For this review, take the finished solid that the model builds, in its own axes (mm). A direction names the side the tool comes from. Coordinates: 2 decimals unless noted, no trailing zeros.
from build123d import *

# Parameters (mm, degrees)
F1_DEPTH     = 7
F2_T2_ANGLE  = 96.7405372454
F2_T4_ANGLE  = 266.8582437325
F2_T6_ANGLE  = 95.969109219
F2_T8_ANGLE  = 264.3512540772
F2_T10_ANGLE = 268.0965177518
F2_T12_ANGLE = 96.2209043171
F2_T14_ANGLE = 96.2209043171
F2_T16_ANGLE = 264.3512540772
F2_T18_ANGLE = 95.969109219
F2_T20_ANGLE = 266.8582437325
F2_T22_ANGLE = 96.7405372454
F2_T24_ANGLE = 268.0965177518


# Not quite as in the source:
# - a fillet or chamfer that OpenCascade refuses, or shapes differently, is made with other operations: its cross-section is extruded or revolved along the edge and cut away or added


with BuildPart() as f1:
    # F0 (on Front) → F1 (new body)
    with BuildSketch(Plane.XZ):
        with BuildLine():
            Line((-28.60048896, 16.5125), (-32.04293994, 18.5))
            ThreePointArc((-32.04293994, 18.5), (-36.2110940276, 7.5997808734), (-36.7769641036, -4.0564653732))
            ThreePointArc((-36.7769641036, -4.0564653732), (-33.6399342951, -1.6712337769), (-29.9995629467, -0.1619351868))
            ThreePointArc((-29.9995629467, -0.1619351868), (-29.5180509711, 5.3558068364), (-28.030388979, 10.6909912395))
            ThreePointArc((-28.030388979, 10.6909912395), (-29.2497876853, 13.5102449097), (-28.60048896, 16.5125))
        make_face()
        with BuildLine():
            ThreePointArc((-28.030388979, 10.6909912395), (-29.5180509711, 5.3558068364), (-29.9995629467, -0.1619351868))
            ThreePointArc((-29.9995629467, -0.1619351868), (-20.1170678219, -0.7895806962), (-12.6676409298, -7.3136659008))
            Line((-12.6676409298, -7.3136659008), (-9.5479300767, -5.5125))
            ThreePointArc((-9.5479300767, -5.5125), (-11.025, 0), (-9.5479300767, 5.5125))
            Line((-9.5479300767, 5.5125), (-19.8969336519, 11.4875))
            ThreePointArc((-19.8969336519, 11.4875), (-23.7589562157, 8.9989236207), (-28.030388979, 10.6909912395))
        make_face()
        with BuildLine():
            ThreePointArc((0, 14.7547752324), (-9.310283358, 17.9279039927), (-14.7448970108, 26.1263853631))
            ThreePointArc((-14.7448970108, 26.1263853631), (-19.3469694385, 22.9280346638), (-23.2738644946, 18.9295333141))
            ThreePointArc((-23.2738644946, 18.9295333141), (-20.3661071395, 17.1899858756), (-19.223711306, 14))
            ThreePointArc((-19.223711306, 14), (-19.3949340289, 12.6994342984), (-19.8969336519, 11.4875))
            Line((-19.8969336519, 11.4875), (-9.5479300767, 5.5125))
            ThreePointArc((-9.5479300767, 5.5125), (-5.5125, 9.5479300767), (0, 11.025))
            Line((0, 11.025), (0, 14.7547752324))
        make_face()
        with BuildLine():
            ThreePointArc((-14.7448970108, 26.1263853631), (-15.2451824532, 30.0359191128), (-14.726480194, 33.9430520298))
            ThreePointArc((-14.726480194, 33.9430520298), (-24.6265431784, 27.6140067915), (-32.04293994, 18.5))
            Line((-32.04293994, 18.5), (-28.60048896, 16.5125))
            ThreePointArc((-28.60048896, 16.5125), (-26.3251091458, 18.5759367359), (-23.2738644946, 18.9295333141))
            ThreePointArc((-23.2738644946, 18.9295333141), (-19.3469694385, 22.9280346638), (-14.7448970108, 26.1263853631))
        make_face()
        with BuildLine():
            ThreePointArc((19.8969336519, 11.4875), (19.6727745701, 16.0763978398), (23.2738644946, 18.9295333141))
            ThreePointArc((23.2738644946, 18.9295333141), (19.3469694385, 22.9280346638), (14.7448970108, 26.1263853631))
            ThreePointArc((14.7448970108, 26.1263853631), (9.310283358, 17.9279039927), (0, 14.7547752324))
            Line((0, 14.7547752324), (0, 11.025))
            ThreePointArc((0, 11.025), (5.5125, 9.5479300767), (9.5479300767, 5.5125))
            Line((9.5479300767, 5.5125), (19.8969336519, 11.4875))
        make_face()
        with BuildLine():
            Line((28.60048896, 16.5125), (32.04293994, 18.5))
            ThreePointArc((32.04293994, 18.5), (24.6265431784, 27.6140067915), (14.726480194, 33.9430520298))
            ThreePointArc((14.726480194, 33.9430520298), (15.1149822826, 31.9885142218), (15.2452247676, 30))
            ThreePointArc((15.2452247676, 30), (15.1196254471, 28.0471035473), (14.7448970108, 26.1263853631))
            ThreePointArc((14.7448970108, 26.1263853631), (19.3469694385, 22.9280346638), (23.2738644946, 18.9295333141))
            ThreePointArc((23.2738644946, 18.9295333141), (26.3251091458, 18.5759367359), (28.60048896, 16.5125))
        make_face()
        with BuildLine():
            ThreePointArc((36.8122346311, -3.7228190211), (36.9530288431, -1.8637755563), (37, 0))
            ThreePointArc((37, 0), (35.7392555727, 9.5763046688), (32.04293994, 18.5))
            Line((32.04293994, 18.5), (28.60048896, 16.5125))
            ThreePointArc((28.60048896, 16.5125), (29.1024885831, 15.3005657016), (29.273711306, 14))
            ThreePointArc((29.273711306, 14), (28.9526221952, 12.2325590968), (28.030388979, 10.6909912395))
            ThreePointArc((28.030388979, 10.6909912395), (29.4933804082, 5.4900375314), (29.9997945679, 0.1110219992))
            ThreePointArc((29.9997945679, 0.1110219992), (33.6494620505, -1.3733111503), (36.8122346311, -3.7228190211))
        make_face()
        with BuildLine():
            ThreePointArc((12.4392811828, -7.1818223394), (19.983625223, -0.5594336383), (29.9997945679, 0.1110219992))
            ThreePointArc((29.9997945679, 0.1110219992), (29.4933804082, 5.4900375314), (28.030388979, 10.6909912395))
            ThreePointArc((28.030388979, 10.6909912395), (23.7589562157, 8.9989236207), (19.8969336519, 11.4875))
            Line((19.8969336519, 11.4875), (9.5479300767, 5.5125))
            ThreePointArc((9.5479300767, 5.5125), (10.6493322348, 2.8534799723), (11.025, 0))
            ThreePointArc((11.025, 0), (10.6493322348, -2.8534799723), (9.5479300767, -5.5125))
            Line((9.5479300767, -5.5125), (12.4392811828, -7.1818223394))
        make_face()
        with BuildLine():
            ThreePointArc((4.7565244845, -29.6205245536), (9.9921782342, -28.2870354427), (14.9037494122, -26.0360952037))
            ThreePointArc((14.9037494122, -26.0360952037), (10.476296354, -17.0266102837), (12.4392811828, -7.1818223394))
            Line((12.4392811828, -7.1818223394), (9.5479300767, -5.5125))
            ThreePointArc((9.5479300767, -5.5125), (5.5125, -9.5479300767), (0, -11.025))
            Line((0, -11.025), (0, -22.975))
            ThreePointArc((0, -22.975), (3.5532115755, -24.4467884245), (5.025, -28))
            ThreePointArc((5.025, -28), (4.9574267788, -28.8213067227), (4.7565244845, -29.6205245536))
        make_face()
        with BuildLine():
            ThreePointArc((-10.6080939152, -15), (-11.7862202639, -20.9020258568), (-15.1400214589, -25.8994160209))
            ThreePointArc((-15.1400214589, -25.8994160209), (-10.1207607074, -28.2412854294), (-4.7565244845, -29.6205245536))
            ThreePointArc((-4.7565244845, -29.6205245536), (-4.0861816456, -25.0753214605), (0, -22.975))
            Line((0, -22.975), (0, -11.025))
            ThreePointArc((0, -11.025), (-5.5125, -9.5479300767), (-9.5479300767, -5.5125))
            Line((-9.5479300767, -5.5125), (-12.6676409298, -7.3136659008))
            ThreePointArc((-12.6676409298, -7.3136659008), (-11.1319048818, -11.0212606962), (-10.6080939152, -15))
        make_face()
        with BuildLine():
            ThreePointArc((-21.9014841146, -29.8215525011), (-11.5239437142, -35.1596177634), (0, -37))
            Line((0, -37), (0, -33.025))
            ThreePointArc((0, -33.025), (-2.9246785395, -32.0861816456), (-4.7565244845, -29.6205245536))
            ThreePointArc((-4.7565244845, -29.6205245536), (-10.1207607074, -28.2412854294), (-15.1400214589, -25.8994160209))
            ThreePointArc((-15.1400214589, -25.8994160209), (-18.267298054, -28.2974207927), (-21.9014841146, -29.8215525011))
        make_face()
        with BuildLine():
            ThreePointArc((0, -37), (11.3644165831, -35.2115043093), (21.6301731615, -30.0189208501))
            ThreePointArc((21.6301731615, -30.0189208501), (18.0140533687, -28.4546333842), (14.9037494122, -26.0360952037))
            ThreePointArc((14.9037494122, -26.0360952037), (9.9921782342, -28.2870354427), (4.7565244845, -29.6205245536))
            ThreePointArc((4.7565244845, -29.6205245536), (2.9246785395, -32.0861816456), (0, -33.025))
            Line((0, -33.025), (0, -37))
        make_face()
    extrude(amount=F1_DEPTH)

    # F2: chamfer of 3 on 12 edges, made by hand

    # F2_s1 → F2_t2 (revolve, cut)
    with BuildSketch(Plane(origin=(0, 0, 0), x_dir=(0, 1, 0), z_dir=(0.9799112872, 0, 0.199433872))):
        Polygon((-4, 37), (-7, 34), (-7, 37), align=None)
    revolve(axis=Axis((0, -7, 0), (0, -1, 0)), revolution_arc=F2_T2_ANGLE, mode=Mode.SUBTRACT)

    # F2_s3 → F2_t4 (revolve, cut)
    with BuildSketch(Plane(origin=(-6.2136111397, 0, -20.8819053013), x_dir=(0, 1, 0), z_dir=(-0.2852012416, 0, -0.9584676582))):
        Polygon((-4, -35.9963697961), (-7, -38.9963697961), (-7, -35.9963697961), align=None)
    revolve(axis=Axis((-25.9807621135, -7, -15), (0, 1, 0)), revolution_arc=F2_T4_ANGLE, mode=Mode.SUBTRACT)

    # F2_s5 → F2_t6 (revolve, cut)
    with BuildSketch(Plane(origin=(0, 0, 0), x_dir=(0, 1, 0), z_dir=(-0.6659555398, 0, 0.7459914336))):
        Polygon((-4, 37), (-7, 34), (-7, 37), align=None)
    revolve(axis=Axis((0, -7, 0), (0, -1, 0)), revolution_arc=F2_T6_ANGLE, mode=Mode.SUBTRACT)

    # F2_s7 → F2_t8 (revolve, cut)
    with BuildSketch(Plane(origin=(21.7325989573, 0, 4.6890781514), x_dir=(0, 1, 0), z_dir=(0.977505701, 0, 0.2109089959))):
        Polygon((-4, -35.7785172869), (-7, -38.7785172869), (-7, -35.7785172869), align=None)
    revolve(axis=Axis((25.9807621135, -7, -15), (0, 1, 0)), revolution_arc=F2_T8_ANGLE, mode=Mode.SUBTRACT)

    # F2_s9 → F2_t10 (revolve, cut)
    with BuildSketch(Plane(origin=(-14.9917229855, 0, 15.4982388241), x_dir=(0, 1, 0), z_dir=(-0.6952640068, 0, 0.718754451))):
        Polygon((-4, -36.1031449725), (-7, -39.1031449725), (-7, -36.1031449725), align=None)
    revolve(axis=Axis((0, -7, 30), (0, 1, 0)), revolution_arc=F2_T10_ANGLE, mode=Mode.SUBTRACT)

    # F2_s11 → F2_t12 (revolve, cut)
    with BuildSketch(Plane(origin=(0, 0, 0), x_dir=(0, 1, 0), z_dir=(-0.3044454567, 0, -0.9525297706))):
        Polygon((-4, 37), (-7, 34), (-7, 37), align=None)
    revolve(axis=Axis((0, -7, 0), (0, -1, 0)), revolution_arc=F2_T12_ANGLE, mode=Mode.SUBTRACT)

    # F2_s13 → F2_t14 (revolve, cut)
    with BuildSketch(Plane(origin=(0, 0, 0), x_dir=(0, 1, 0), z_dir=(-0.3044454567, 0, -0.9525297706))):
        Polygon((-3, 37), (0, 34), (0, 37), align=None)
    revolve(axis=Axis((0, 0, 0), (0, -1, 0)), revolution_arc=F2_T14_ANGLE, mode=Mode.SUBTRACT)

    # F2_s15 → F2_t16 (revolve, cut)
    with BuildSketch(Plane(origin=(21.7325989573, 0, 4.6890781514), x_dir=(0, 1, 0), z_dir=(0.977505701, 0, 0.2109089959))):
        Polygon((-3, -35.7785172869), (0, -38.7785172869), (0, -35.7785172869), align=None)
    revolve(axis=Axis((25.9807621135, 0, -15), (0, 1, 0)), revolution_arc=F2_T16_ANGLE, mode=Mode.SUBTRACT)

    # F2_s17 → F2_t18 (revolve, cut)
    with BuildSketch(Plane(origin=(0, 0, 0), x_dir=(0, 1, 0), z_dir=(-0.6659555398, 0, 0.7459914336))):
        Polygon((-3, 37), (0, 34), (0, 37), align=None)
    revolve(axis=Axis((0, 0, 0), (0, -1, 0)), revolution_arc=F2_T18_ANGLE, mode=Mode.SUBTRACT)

    # F2_s19 → F2_t20 (revolve, cut)
    with BuildSketch(Plane(origin=(-6.2136111397, 0, -20.8819053013), x_dir=(0, 1, 0), z_dir=(-0.2852012416, 0, -0.9584676582))):
        Polygon((-3, -35.9963697961), (0, -38.9963697961), (0, -35.9963697961), align=None)
    revolve(axis=Axis((-25.9807621135, 0, -15), (0, 1, 0)), revolution_arc=F2_T20_ANGLE, mode=Mode.SUBTRACT)

    # F2_s21 → F2_t22 (revolve, cut)
    with BuildSketch(Plane(origin=(0, 0, 0), x_dir=(0, 1, 0), z_dir=(0.9799112872, 0, 0.199433872))):
        Polygon((-3, 37), (0, 34), (0, 37), align=None)
    revolve(axis=Axis((0, 0, 0), (0, -1, 0)), revolution_arc=F2_T22_ANGLE, mode=Mode.SUBTRACT)

    # F2_s23 → F2_t24 (revolve, cut)
    with BuildSketch(Plane(origin=(-14.9917229855, 0, 15.4982388241), x_dir=(0, 1, 0), z_dir=(-0.6952640068, 0, 0.718754451))):
        Polygon((-3, -36.1031449725), (0, -39.1031449725), (0, -36.1031449725), align=None)
    revolve(axis=Axis((0, 0, 30), (0, 1, 0)), revolution_arc=F2_T24_ANGLE, mode=Mode.SUBTRACT)


solid = f1.part
1. Take a section at A-A, the plane y = -1.5. Give the number of separate pieces and of enclosed holes in the cut face, plus the area to 3 significant figures.
Answer below:
separate pieces: 1
enclosed holes: 4
area: 1,570 mm2
2. To check wall thickness, follow L1, parallel to X at y = -2.25, z = 16; L2, parallel to Z at x = -1, y = -3.5; L3, parallel to X at y = -4, z = -1.5. State the ranges of each line that lie inside material, in increasing order.
Answer below:
L1: x = -32.53 to -28.86, -19.64 to -7.74, 7.74 to 19.64, 28.86 to 32.53
L2: z = -36.99 to -32.92, -23.08 to -10.98, 10.98 to 14.79
L3: x = -36.97 to -33.33, -18.63 to -10.92, 10.92 to 18.09, 33.87 to 36.97
3. The part is to be moulded in two halves that separate along X. For faces 1 (the face through (0, -6, -35)), 2 (the face through (-29.95, -0.81, 17.74)), 3 (the face through (-12.708, -2.812, -6.878)), say which applies: +X half, -X half, draft (parallel to the pull), parting line (faces both ways), or undercut.
Answer below:
face 1: parting line
face 2: -X half
face 3: undercut
4. Machinability: for faces 4 (the face through (0.4, -2.81, 14.57)), 5 (the face through (0, -1, -35)), which of the approach directions +Z, -Z, +X, -X, +Y, -Y give a long, thin tool a straight path to every point of the face, cutting with its end or side? Answer none if there is none.
Answer below:
face 4: +Y
face 5: -Z, +Y
5. Clearance check with flat-ended pins moving along their axes: pin 1 Ø3 at (y, z) = (-5, 6) entering from -X; pin 2 Ø1 at (x, y) = (28.5, -3) entering from -Z; pin 3 Ø2 at (x, y) = (-26.5, -2) entering from +Z. State where each tip first meets the part, or that it passes through.
Answer below:
pin 1: stops at x = -36.68
pin 2: stops at z = 0.34
pin 3: stops at z = 26.14
